from build123d import *

# Parameters (mm, degrees)
BOSS_EXTRUDE1_DEPTH = 14
SKETCH3_R           = 2.469718116
CUT_EXTRUDE1_DEPTH  = 21


with BuildPart() as part:
    # Sketch1 → Boss-Extrude1 (new body)
    with BuildSketch(Plane(origin=(0, 0, 0), x_dir=(1, 0, 0), z_dir=(0, 1, 0))):
        with BuildLine():
            Line((8, 67.50149873), (8, 79.954057008))
            add(Edge.make_bspline(
                [(0, 45), (-4.267413412, 52.702157849), (-3.849710429, 67.232110416), (4.572220088, 77.524864833), (8, 79.954057008)],
                knots=[0, 0, 0, 0, 0.616858973, 0.90735247, 0.90735247, 0.90735247, 0.90735247], degree=3))
            Line((0, 45), (0, 15))
            Line((0, 15), (60, 15))
            Line((60, 15), (60, 45))
            add(Edge.make_bspline(
                [(60, 45), (64.267413412, 52.702157849), (63.849710429, 67.232110416), (55.427779912, 77.524864833), (52, 79.954057008)],
                knots=[0, 0, 0, 0, 0.616858973, 0.90735247, 0.90735247, 0.90735247, 0.90735247], degree=3))
            Line((52, 79.954057008), (52, 70.29729534))
            Line((52, 70.29729534), (52, 28))
            Line((52, 28), (8, 28))
            Line((8, 28), (8, 67.50149873))
        make_face()
    extrude(amount=BOSS_EXTRUDE1_DEPTH)

    # Sketch3 → Cut-Extrude1 (cut)
    with BuildSketch(Plane.XZ):
        with Locations(Location((30, -20, 0), (0, 0, 270))):
            Circle(SKETCH3_R)
    extrude(amount=-CUT_EXTRUDE1_DEPTH, mode=Mode.SUBTRACT)


solid = part.part
Verification items for the finished model (mm, model axes). A direction names the side the tool comes from. Give positions to 0.01 mm unless a question says otherwise; leave off trailing zeros. Write each loop counter-clockwise with the first axis right and the second up, starting at its lowest first coordinate (ties: lowest second). Pieces come first, ordered by that corner, then holes. Notation, with made-up numbers: (-31, -11.5) -> (18, -11.5) arc R20 ccw to (18, 22.5) -> close; hole circle Ø10 at (64, 67.5). An arc over 180 degrees is marked (long way). Use CSV: the item, a comma, the result in double quotes.
(1) Sectioned sample at B-B (x = 30). Record the cut outline in (y, z), plus the area to 3 significant figures.
Derived:
outline,"(0, -28) -> (14, -28) -> (14, -22.47) -> (0, -22.47) -> close; (0, -17.53) -> (14, -17.53) -> (14, -15) -> (0, -15) -> close"
area,"113 mm^2"
(2) Release check for a two-part mould opening along Z. For faces 1 (the flat face through (52, 7, -54)), 2 (the cylindrical face through (32.45, 6.9, -19.68)), 3 (the flat face through (30, 7, -28)) record: +Z half, -Z half, draft (parallel to the pull), parting line (faces both ways), or undercut.
Derived:
face 1,"draft"
face 2,"undercut"
face 3,"-Z half"
(3) Set-up check for faces 4 (the flat face through (8, 7, -54)), 5 (the flat face through (23, 0, -26)), 6 (the flat face through (23, 14, -26)), 7 (the flat face through (60, 7, -30)), 8 (the flat face through (0, 7, -30)): record each of +Z, -Z, +X, -X, +Y, -Y from which the full face is reachable in a straight line by a thin tool's end or side.
Derived:
face 4,"-Z, +Y, -Y"
face 5,"+Z, -Z, +X, -X, -Y"
face 6,"+Z, -Z, +X, -X, +Y"
face 7,"+Z, +X, +Y, -Y"
face 8,"+Z, -X, +Y, -Y"
(4) Sectioned sample at C-C (x = 18). Record the cut outline in (y, z).
Derived:
outline,"(0, -28) -> (14, -28) -> (14, -15) -> (0, -15) -> close"
(5) Material ranges on L1, parallel to X at y = 5, z = -20; L2, parallel to X at y = 1.5, z = -37; L3, parallel to Z at x = 12, y = 6.5, recorded low to high.
Derived:
L1,"x = 0 to 27.53, 32.47 to 60"
L2,"x = 0 to 8, 52 to 60"
L3,"z = -28 to -15"
(6) Go/stop test with flat-tipped pins: pin 1 (3 mm diameter, centred on y = 6, z = -65, fed in from -X); pin 2 (7 mm diameter, centred on y = 8, z = -42, fed in from -X); pin 3 (6 mm diameter, centred on y = 7, z = -28, fed in from +X). Record where each tip stops, or that it passes through.
Derived:
pin 1,"stops at x = -2.45"
pin 2,"stops at x = -0.27"
pin 3,"stops at x = 60"
(7) Sectioned sample at A-A (z = -20). Record the cut outline in (x, y).
Derived:
outline,"(0, 0) -> (27.53, 0) -> (27.53, 14) -> (0, 14) -> close; (32.47, 0) -> (60, 0) -> (60, 14) -> (32.47, 14) -> close"
